from build123d import *

# Parameters (mm, degrees)
SKETCH1_W           = 4
SKETCH1_H           = 27.5
SKETCH2_R           = 10
BOSS_EXTRUDE1_DEPTH = 1
SKETCH3_R           = 9.5
BOSS_EXTRUDE2_DEPTH = 8.1
SKETCH4_R           = 8.5
BOSS_EXTRUDE3_DEPTH = 12.2
CUT_EXTRUDE1_DEPTH  = 19.5
HOLE1_D             = 5
HOLE1_DEPTH         = 25.3
HOLE1_CBORE_D       = 9
HOLE1_CBORE_DEPTH   = 10
CHAMFER1_SIZE       = 0.5
FILLET1_R           = 1
FILLET2_R           = 4


with BuildPart() as part:
    # Sketch1 → Revolve1 (revolve)
    with BuildSketch(Plane(origin=(0, 0, 216.5), x_dir=(-1, 0, 0), z_dir=(0, 0, -1)), mode=Mode.PRIVATE) as revolve1_sk:
        with Locations((-182.6, -12.75)):
            Rectangle(SKETCH1_W, SKETCH1_H)
    revolve(revolve1_sk.sketch.rotate(Axis((184.6, -26.5, 216.5), (-1, 0, 0)), 270), axis=Axis((184.6, -26.5, 216.5), (-1, 0, 0)))

    # Sketch2 → Boss-Extrude1 (add)
    with BuildSketch(Plane(origin=(184.6, 0, 0), x_dir=(0, 0, -1), z_dir=(1, 0, 0))):
        with Locations((-216.5, -26.5)):
            Circle(SKETCH2_R)
    extrude(amount=BOSS_EXTRUDE1_DEPTH)

    # Sketch3 → Boss-Extrude2 (add)
    with BuildSketch(Plane.ZY.offset(-180.6)):
        with Locations((216.5, -26.5)):
            Circle(SKETCH3_R)
    extrude(amount=BOSS_EXTRUDE2_DEPTH)

    # Sketch4 → Boss-Extrude3 (add)
    with BuildSketch(Plane.ZY.offset(-172.5)):
        with Locations((216.5, -26.5)):
            Circle(SKETCH4_R)
    extrude(amount=BOSS_EXTRUDE3_DEPTH)

    # Sketch5 → Cut-Extrude1 (cut)
    with BuildSketch(Plane.ZY.offset(-160.3)):
        with BuildLine():
            Line((220.906082937, -25.249228687), (217.750771313, -22.093917063))
            ThreePointArc((217.750771313, -22.093917063), (216.434925146, -20.269610576), (214.788393439, -21.802085252))
            ThreePointArc((214.788393439, -21.802085252), (212.964466094, -30.035533906), (221.197914748, -28.211606561))
            ThreePointArc((221.197914748, -28.211606561), (222.730389424, -26.565074854), (220.906082937, -25.249228687))
        make_face()
    extrude(amount=-CUT_EXTRUDE1_DEPTH, mode=Mode.SUBTRACT)

    # Hole1
    with Locations(Plane(origin=(185.6, 0, 0), x_dir=(0, 0, -1), z_dir=(1, 0, 0))):
        with Locations((-216.5, -26.5)):
            CounterBoreHole(HOLE1_D / 2, HOLE1_CBORE_D / 2, HOLE1_CBORE_DEPTH, depth=HOLE1_DEPTH)

    # Chamfer1
    chamfer1_edges = [part.edges().sort_by_distance(p)[0] for p in [
        (160.3, -26.5, 208),
        (180.6, -26.5, 189),
        (185.6, -26.5, 221),
        (184.6, -26.5, 189),
    ]]
    chamfer(chamfer1_edges, length=CHAMFER1_SIZE)

    # Fillet1
    # the kernel refuses this fillet: 1 mm, written as the material it takes off along each edge
    with BuildSketch(Plane(origin=(159.134806492, -25.249228687, 220.906082937), x_dir=(0, 0.7071067811864904, -0.7071067811866047), z_dir=(1, 0, 0))) as fillet1_piece_1:
        with BuildLine():
            CenterArc((0.466077403, 1), FILLET1_R, 226.054480438, 43.945519562)
            ThreePointArc((-0.22789666, 0.28), (-0.105493762, 0.146881314), (0, 0))
            Line((0, 0), (0.466077403, 0))
        make_face()
    extrude(amount=20.665193508, mode=Mode.SUBTRACT)
    with BuildSketch(Plane(origin=(159.134806492, -22.093917063, 217.750771313), x_dir=(0, -0.7071067811865017, 0.7071067811865932), z_dir=(1, 0, 0))) as fillet1_piece_2:
        with BuildLine():
            CenterArc((0.466077403, -1), FILLET1_R, 90, 43.945519562)
            ThreePointArc((-0.22789666, -0.28), (-0.105493762, -0.146881314), (0, 0))
            Line((0, 0), (0.466077403, 0))
        make_face()
    extrude(amount=20.665193508, mode=Mode.SUBTRACT)
    with BuildSketch(Plane(origin=(159.010183368, -28.211606561, 221.197914748), x_dir=(0, -0.9206703550954229, -0.39034100123925997), z_dir=(1, 0, 0))) as fillet1_piece_3:
        with BuildLine():
            CenterArc((0.567519318, -0.998668212), FILLET1_R, 92.957354948, 48.80173568)
            ThreePointArc((-0.217895829, -0.37969887), (-0.095021383, -0.197841382), (0, 0))
            ThreePointArc((0, 0), (0.257963326, -0.006658942), (0.515926653, 0))
        make_face()
    extrude(amount=20.789816632, mode=Mode.SUBTRACT)
    with BuildSketch(Plane(origin=(159.010183368, -21.802085252, 214.788393439), x_dir=(0, -0.3903410012394471, -0.9206703550953437), z_dir=(1, 0, 0))) as fillet1_piece_4:
        with BuildLine():
            CenterArc((0.567519318, 0.998668212), FILLET1_R, 218.240909372, 48.80173568)
            ThreePointArc((-0.217895829, 0.37969887), (-0.095021383, 0.197841382), (0, 0))
            ThreePointArc((0, 0), (0.257963326, 0.006658942), (0.515926653, 0))
        make_face()
    extrude(amount=20.789816632, mode=Mode.SUBTRACT)

    # Fillet2
    fillet2_edges = [part.edges().sort_by_distance(p)[0] for p in [
        (180.6, -26.5, 207),
    ]]
    fillet(fillet2_edges, radius=FILLET2_R)


solid = part.part
Can you work these out from the model? Positions are in its coordinate system, mm. A direction names the side the tool comes from. Round coordinates to 2 decimals unless told otherwise and drop trailing zeros. Order: outer loops, then holes, each group sorted by start corner. A loop starts at its lowest first (then second) coordinate and runs counter-clockwise, first axis right, second up. Notation, with made-up numbers: M 73,-27 L 102,-27 A6 ccw 102,-18 Z; hole C -32,-15.75 d6. An arc over 180 degrees is marked long. Use a Markdown table: item, result.
1) If we mould it in two halves opening along Y, with no side actions, what happens to faces 1 (the face through (160.3, -32, 216)), 2 (the face through (166.73, -26.13, 208.01)), 3 (the face through (175.6, -23, 219))? For each: +Y half, -Y half, draft (parallel to the pull), parting line (faces both ways), or undercut.
Geometry says:
| item | result |
|---|---|
| face 1 | draft |
| face 2 | parting line |
| face 3 | undercut |
2) Imagine slicing it at D-D (x = 177.5). List the corners of the cut face in (y, z) for me.
Geometry says:
| item | result |
|---|---|
| outline | C -26.5,216.5 d19.21; hole M -28.69,221 A5 ccw long -22,214.31 A1 cw -21.37,214.84 A1.5 ccw -21.73,217.79 A1 cw -22.23,217.93 A4.5 ccw -25.07,220.77 A1 cw -25.21,221.27 A1.5 ccw -28.16,221.63 A1 cw Z |
3) Imagine slicing it at A-A (x = 168.75). List the corners of the cut face in (y, z) for me, then the cut area to 3 significant figures.
Geometry says:
| item | result |
|---|---|
| outline | C -26.5,216.5 d17; hole M -28.69,221 A5 ccw long -22,214.31 A1 cw -21.37,214.84 A1.5 ccw -21.73,217.79 A1 cw -22.42,218.08 L -24.92,220.58 A1 cw -25.21,221.27 A1.5 ccw -28.16,221.63 A1 cw Z |
| area | 146 mm² |
4) On a 3-axis mill with a long thin cutter (end or side, diameter ignored), from which of +Z, -Z, +X, -X, +Y, -Y can I reach the whole of each face in a straight line? I mean faces 4 (the face through (169.91, -29.94, 212.87)), 5 (the face through (185.6, -24.1, 221.1)), 6 (the face through (185.093, -30.33, 207.263)), 7 (the face through (167.843, -23.689, 219.346)). Say none if no direction works.
Geometry says:
| item | result |
|---|---|
| face 4 | -X |
| face 5 | +Z, -Z, +X, +Y, -Y |
| face 6 | +X |
| face 7 | +X, -X |
5) I'm going to push flat-ended pins straight in: P1, Ø1.5, axis at y = -29.5, z = 202.5, coming from the +X side; P2, Ø3, axis at x = 176.5, z = 213.5, coming from the +Y side; P3, Ø4, axis at y = -37, z = 228.5, coming from the -X side. Where does each tip first touch, or does it pass through?
Geometry says:
| item | result |
|---|---|
| P1 | stops at x = 184.6 |
| P2 | stops at y = -17.08 |
| P3 | stops at x = 180.6 |
6) If I drill on line 1 along Y through (x, z) = (164.75, 216.5); line 2 along X through (y, z) = (-3, 221.5); line 3 along Y through (x, z) = (178.5, 216.5), over which ranges is the centre line in solid material (lowest first)?
Geometry says:
| item | result |
|---|---|
| line 1 | y = -35 to -31.5, -20.28 to -18 |
| line 2 | x = 180.6 to 184.6 |
| line 3 | y = -36.48 to -31.5, -20.28 to -16.52 |
